Can you work these out from the drawing? Everything is in mm from the part's minimum corner. Round coordinates to 2 decimals unless told otherwise and drop trailing zeros. Order: outer loops, then holes, each group sorted by start corner. A loop starts at its lowest first (then second) coordinate and runs counter-clockwise, first axis right, second up. Notation, with made-up numbers: (-24, 55.25) - (10, 55.25) arc R22 cw to (10, 91.25) - close; hole circle Ø1 at (68, 42.25). An arc over 180 degrees is marked (long way). Write item = value, one per line.
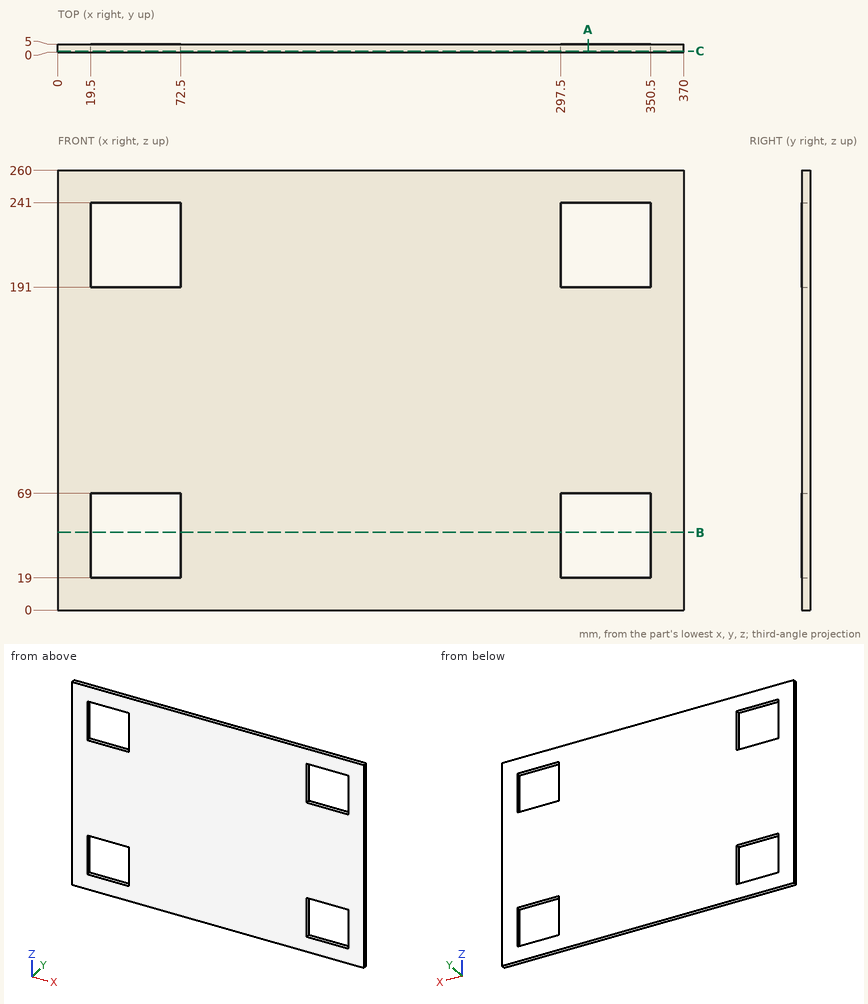
(1) If we section it at B-B (z = 46): Write out the boundary of the cut face in (x, y).
Computed:
outline = (0, 0) - (19.5, 0) - (19.5, 5) - (0, 5) - close; (72.5, 0) - (297.5, 0) - (297.5, 5) - (72.5, 5) - close; (350.5, 0) - (370, 0) - (370, 5) - (350.5, 5) - close
(2) If we section it at A-A (x = 313.5): Write out the boundary of the cut face in (y, z).
Computed:
outline = (0, 0) - (5, 0) - (5, 19) - (0, 19) - close; (0, 69) - (5, 69) - (5, 191) - (0, 191) - close; (0, 241) - (5, 241) - (5, 260) - (0, 260) - close
(3) If I drill on line 1 (X direction, y = 4.75, z = 24); line 2 (Z direction, x = 56, y = 3), over which ranges is the centre line in solid material (lowest first)? Write a range as from..to.
Computed:
line_1 = 0..19.5, 72.5..297.5, 350.5..370
line_2 = 0..19, 69..191, 241..260
(4) If we section it at C-C (y = 0.85): Write out the boundary of the cut face in (x, z), plus the area to 3 significant figures.
Computed:
outline = (0, 0) - (370, 0) - (370, 260) - (0, 260) - close; hole (19.5, 19) - (72.5, 19) - (72.5, 69) - (19.5, 69) - close; hole (19.5, 191) - (72.5, 191) - (72.5, 241) - (19.5, 241) - close; hole (297.5, 19) - (350.5, 19) - (350.5, 69) - (297.5, 69) - close; hole (297.5, 191) - (350.5, 191) - (350.5, 241) - (297.5, 241) - close
area = 85,600 mm^2
